Can you work these out from the model? Positions are in its coordinate system, mm. Give positions to 0.01 mm unless a question says otherwise; leave off trailing zeros. Order: outer loops, then holes, each group sorted by start corner. A loop starts at its lowest first (then second) coordinate and runs counter-clockwise, first axis right, second up. Notation, with made-up numbers: (38.5, 29.25) - (63.5, 29.25) arc R9 ccw to (63.5, 33.25) - close; hole circle Ø3 at (70.25, -11.5). An arc over 180 degrees is marked (long way). One line per question, with ' | ' between items.
```python
from build123d import *

# Parameters (mm, degrees)
BOSS_EXTRUDE1_DEPTH = 1828
SKETCH2_W           = 67.392754287
SKETCH2_H           = 36.940615493
SKETCH2_R           = 2.5
BOSS_EXTRUDE2_DEPTH = 5


with BuildPart() as part:
    # Sketch1 → Boss-Extrude1 (new body)
    with BuildSketch(Plane.XY):
        Polygon((-20.987492455, 6.600745666), (-15.987492455, 6.600745666), (-15.987492455, -2.358820079), (19.012507545, -2.358820079), (19.012507545, 6.600745666), (24.012507545, 6.600745666), (24.012507545, -14.726832534), (-20.987492455, -14.726832534), align=None)
    extrude(amount=BOSS_EXTRUDE1_DEPTH)

    # Sketch2 → Boss-Extrude2 (add)
    with BuildSketch(Plane(origin=(0, 0, 0), x_dir=(-1, 0, 0), z_dir=(0, 0, -1))):
        with Locations((1.099137048, 0.254222391)):
            Rectangle(SKETCH2_W, SKETCH2_H)
        with Locations((-27.597240096, 13.724530137)):
            Circle(SKETCH2_R, mode=Mode.SUBTRACT)
        with Locations((31.565303785, 13.724530137)):
            Circle(SKETCH2_R, mode=Mode.SUBTRACT)
        with Locations((31.414421828, -13.216085356)):
            Circle(SKETCH2_R, mode=Mode.SUBTRACT)
        with Locations((-27.748122053, -13.216085356)):
            Circle(SKETCH2_R, mode=Mode.SUBTRACT)
    extrude(amount=BOSS_EXTRUDE2_DEPTH)


solid = part.part
```
(1) Will these pins go through, and if not, where does the flat tip stop? pin 1 (22.5 mm diameter, centred on x = 4, z = 1132.5, fed in from -Y); pin 2 (4 mm diameter, centred on x = 21, z = 555.5, fed in from +Y); pin 3 (8 mm diameter, centred on y = -12.5, z = 799.5, fed in from +X).
Answer below:
pin 1: y = -14.73 | pin 2: y = 6.6 | pin 3: x = 24.01
(2) Imagine slicing it at B-B (x = -4.5). List the corners of the cut face in (y, z) for me, and give its area (3 significant figures).
Answer below:
outline: (-18.22, -5) - (18.72, -5) - (18.72, 0) - (-2.36, 0) - (-2.36, 1828) - (-14.73, 1828) - (-14.73, 0) - (-18.22, 0) - close | area: 22,800 mm^2
(3) If I drill on line 1 (X direction, y = 1, z = 1014); line 2 (Y direction, x = -15, z = 432); line 3 (Z direction, x = 16, y = 5.5), over which ranges is the centre line in solid material (lowest first)?
Answer below:
line 1: -20.99 to -15.99, 19.01 to 24.01 | line 2: -14.73 to -2.36 | line 3: -5 to 0
(4) If we mould it in two halves opening along X, with no side actions, what happens to faces 1 (the face through (1, -2.359, 901)), 2 (the face through (2, -14.727, 901))? For each: released by +X, released by -X, zero draft, split by the parting line, or undercut.
Answer below:
face 1: undercut | face 2: zero draft
(5) Imagine slicing it at A-A (z = 763). List the corners of the cut face in (x, y) for me.
Answer below:
outline: (-20.99, -14.73) - (24.01, -14.73) - (24.01, 6.6) - (19.01, 6.6) - (19.01, -2.36) - (-15.99, -2.36) - (-15.99, 6.6) - (-20.99, 6.6) - close
